Design review of the part built by this model. Coordinates are the model's own, in mm. A direction names the side the tool comes from. Give positions to 0.01 mm unless a question says otherwise; leave off trailing zeros. Order: outer loops, then holes, each group sorted by start corner. A loop starts at its lowest first (then second) coordinate and runs counter-clockwise, first axis right, second up. Notation, with made-up numbers: (17.5, -29) -> (70.5, -29) arc R5 ccw to (70.5, -22) -> close; hole circle Ø6 at (12, -39.5). An arc over 180 degrees is marked (long way). One line per item, written item: value.
from build123d import *

# Parameters (mm, degrees)
PAD_DEPTH   = 20
FILLET_R    = 3
FILLET001_R = 2


with BuildPart() as part:
    # Sketch → Pad (new body)
    with BuildSketch(Plane.XZ):
        with BuildLine():
            Line((0, 0), (0, 37))
            Line((0, 37), (3, 44))
            Line((3, 44), (3, 4))
            Line((3, 4), (26, 4))
            Line((26, 4), (21, 34))
            ThreePointArc((23.448856, 44), (21.197055, 39.251589), (21, 34))
            ThreePointArc((25.84203, 42.190943), (25.551614, 44.294231), (23.448856, 44))
            ThreePointArc((25.84203, 42.190943), (24.041555, 38.293355), (24.041381, 34))
            Line((24.041381, 34), (29.708048, 0))
            Line((29.708048, 0), (0, 0))
        make_face()
    extrude(amount=PAD_DEPTH)

    # Fillet
    fillet_edges = [part.edges().sort_by_distance(p)[0] for p in [
        (26, -10, 4),
        (3, -10, 4),
    ]]
    fillet(fillet_edges, radius=FILLET_R)

    # Fillet001
    fillet001_edges = [part.edges().sort_by_distance(p)[0] for p in [
        (0, -10, 0),
        (29.708048, -10, 0),
    ]]
    fillet(fillet001_edges, radius=FILLET001_R)


solid = part.part
Item 1: Add section B-B on z = 39. Give the boundary of the cut face in (x, y).
Returned:
outline: (0.86, -20) -> (3, -20) -> (3, 0) -> (0.86, 0) -> close; (21.14, -20) -> (24.22, -20) -> (24.22, 0) -> (21.14, 0) -> close
Item 2: Add section C-C on x = 22. Give the boundary of the cut face in (y, z).
Returned:
outline: (-20, 0) -> (0, 0) -> (0, 4) -> (-20, 4) -> close; (-20, 28) -> (0, 28) -> (0, 41.56) -> (-20, 41.56) -> close
Item 3: Draft analysis for pull direction Z (two halves, no side actions). For faces 4 (the cylindrical face through (3.86, -10.14, 4.9)), 5 (the flat face through (23.4, 0, 20.8)), 6 (the cylindrical face through (24.72, -10.14, 5.03)), state which applies: pulls with the +Z half, pulls with the -Z half, needs draft (parallel to the pull), parting line crosses it, or undercut.
Returned:
face 4: pulls with the +Z half
face 5: needs draft
face 6: undercut
Item 4: Machinability: for faces 1 (the cylindrical face through (21.215, -9.86, 39.323)), 2 (the flat face through (26.644, -9.86, 18.386)), 3 (the flat face through (3, -10, 26)), which of the approach directions +Z, -Z, +X, -X, +Y, -Y give a long, thin tool a straight path to every point of the face, cutting with its end or side? Answer none if there is none.
Returned:
face 1: +Y, -Y
face 2: +X, +Y, -Y
face 3: +Z, +Y, -Y
Item 5: To check wall thickness, follow line 1 along Z through (x, y) = (7.5, -12.75); line 2 along X through (y, z) = (-11.5, 40.5); line 3 along X through (y, z) = (-18, 24.5). State the ranges of each line that lie inside material, in increasing order. Write a range as from..to.
Returned:
line 1: 0..4
line 2: 1.5..3, 21.57..24.81
line 3: 0..3, 22.58..25.62
Item 6: Add section A-A on y = -10. Give the boundary of the cut face in (x, z), plus the area to 3 significant figures.
Returned:
outline: (0, 2) arc R2 ccw to (2, 0) -> (27.35, 0) arc R2 ccw to (29.32, 2.33) -> (24.04, 34) arc R10 cw to (25.84, 42.19) arc R1.5 ccw to (23.45, 44) arc R13.06 ccw to (21, 34) -> (25.42, 7.49) arc R3 cw to (22.46, 4) -> (6, 4) arc R3 cw to (3, 7) -> (3, 44) -> (0, 37) -> close
area: 353 mm²
Item 7: Add section D-D on x = 7.75. Give the boundary of the cut face in (y, z), plus the area to 3 significant figures.
Returned:
outline: (-20, 0) -> (0, 0) -> (0, 4) -> (-20, 4) -> close
area: 80.0 mm²
Item 8: Clearance check with flat-ended pins moving along their axes: P1, Ø5, axis at x = 12.5, y = -13.5, coming from the +Z side; P2, Ø4, axis at x = 22.5, y = -14, coming from the +Z side; P3, Ø6, axis at y = -7, z = 28, coming from the +X side. State where each tip first meets the part, or that it passes through.
Returned:
P1: z = 4
P2: z = 44.59
P3: x = 25.54
